CAD build for the part. Positions are in the model's coordinates, mm. Face numbers are marked on the shaded views. A direction names the side the tool comes from. Coordinates: 2 decimals unless noted, no trailing zeros. Loops run counter-clockwise (first coordinate to the right, second up) from the corner with the lowest first, then second, coordinate; pieces in that order, holes last. Notation, with made-up numbers: (21.5, 72) - (28.5, 72) arc R12 ccw to (28.5, 76) - close; hole circle Ø10 at (49.5, 56). An arc over 180 degrees is marked (long way). Put each result on its own line as item: value.
```python
from build123d import *

# Parameters (mm, degrees)
SKETCH1_W             = 4.45
SKETCH1_H             = 6
BOSS_EXTRUDE1_DEPTH   = 7.5
BOSS_EXTRUDE1_2_DEPTH = 7.5
SKETCH2_W             = 6.25
SKETCH2_H             = 6
SKETCH2_R             = 1.75
SKETCH2_W_2           = 4.260679938
SKETCH2_W_3           = 0.189320062
SKETCH2_W_4           = 7.55
BOSS_EXTRUDE2_DEPTH   = 3
SKETCH3_W             = 4
SKETCH3_H             = 1
CUT_EXTRUDE1_DEPTH    = 5


with BuildPart() as part:
    # Sketch1 → Boss-Extrude1 (new body)
    with BuildSketch(Plane.XY):
        with Locations((-3.775, -1.877941176)):
            Rectangle(SKETCH1_W, SKETCH1_H)
    extrude(amount=BOSS_EXTRUDE1_DEPTH)



with BuildPart() as body_2:
    # Sketch1 → Boss-Extrude1 2 (new body)
    with BuildSketch(Plane.XY):
        with Locations((3.775, -1.877941176)):
            Rectangle(SKETCH1_W, SKETCH1_H)
    extrude(amount=BOSS_EXTRUDE1_2_DEPTH)


with BuildPart() as part_1:
    add(part.part)

    add(body_2.part)  # Boss-Extrude2 merges body 2
    # Sketch2 → Boss-Extrude2 (add)
    # profile 1 of 5: a face of its own
    with BuildSketch(Plane(origin=(0, 0, 0), x_dir=(-1, 0, 0), z_dir=(0, 0, -1))):
        with Locations((-9.125, -1.877941176)):
            Rectangle(SKETCH2_W, SKETCH2_H)
        with Locations((-9.030339969, -1.877941176)):
            Circle(SKETCH2_R, mode=Mode.SUBTRACT)
    # profile 2 of 5: a face of its own
    with BuildSketch(Plane(origin=(0, 0, 0), x_dir=(-1, 0, 0), z_dir=(0, 0, -1))):
        with Locations((-3.680339969, -1.877941176)):
            Rectangle(SKETCH2_W_2, SKETCH2_H)
    # profile 3 of 5: a face of its own
    with BuildSketch(Plane(origin=(0, 0, 0), x_dir=(-1, 0, 0), z_dir=(0, 0, -1))):
        with Locations((-5.905339969, -1.877941176)):
            Rectangle(SKETCH2_W_3, SKETCH2_H)
    # profile 4 of 5: a face of its own
    with BuildSketch(Plane(origin=(0, 0, 0), x_dir=(-1, 0, 0), z_dir=(0, 0, -1))):
        with Locations((2.225, -1.877941176)):
            Rectangle(SKETCH2_W_4, SKETCH2_H)
    # profile 5 of 5: a face of its own
    with BuildSketch(Plane(origin=(0, 0, 0), x_dir=(-1, 0, 0), z_dir=(0, 0, -1))):
        with Locations((9.125, -1.877941176)):
            Rectangle(SKETCH2_W, SKETCH2_H)
        with Locations((9.030339969, -1.877941176)):
            Circle(SKETCH2_R, mode=Mode.SUBTRACT)
    extrude(amount=BOSS_EXTRUDE2_DEPTH)

    # Sketch3 → Cut-Extrude1 (cut)
    with BuildSketch(Plane.XY.offset(7.5)):
        with Locations((0, -1.877941176)):
            Rectangle(SKETCH3_W, SKETCH3_H)
    extrude(amount=-CUT_EXTRUDE1_DEPTH, mode=Mode.SUBTRACT)


solid = part_1.part
```
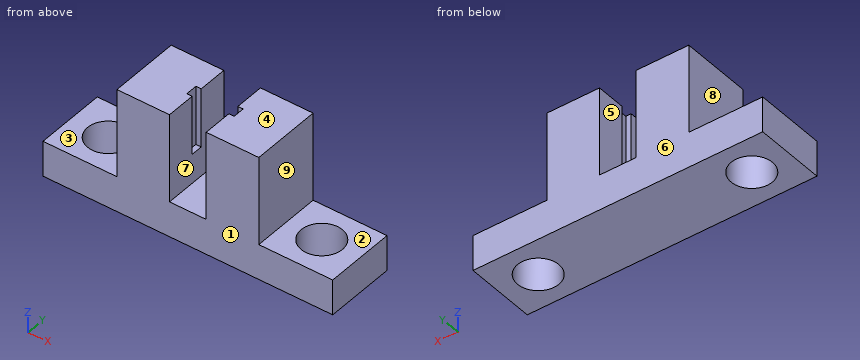
Q1. Slice it at C-C, the plane y = 0.2. Give the cut face in (x, z).
Determined:
outline: (-12.25, -3) - (12.25, -3) - (12.25, 0) - (6, 0) - (6, 7.5) - (1.55, 7.5) - (1.55, 0) - (-1.55, 0) - (-1.55, 7.5) - (-6, 7.5) - (-6, 0) - (-12.25, 0) - close
Q2. Wall check: L1, parallel to X at y = -4.25, z = 1.75; L2, parallel to Y at x = -1.75, z = 6.5; L3, parallel to X at y = -2, z = 3.5. Give the ranges that are in metal, low to high. Write a range as from..to.
Determined:
L1: -6..-1.55, 1.55..6
L2: -4.88..-2.38, -1.38..1.12
L3: -6..-2, 2..6
Q3. Mould opens along X. For the marked faces 6, 7, 8 and 9 say: +X half, -X half, draft (parallel to the pull), parting line (faces both ways), or undercut.
Determined:
face 6: draft
face 7: undercut
face 8: -X half
face 9: +X half
Q4. Slice it at B-B, the plane x = -9. Give the cut face in (y, z), then the cut area to 3 significant figures.
Determined:
outline: (-4.88, -3) - (-3.63, -3) - (-3.63, 0) - (-4.88, 0) - close; (-0.13, -3) - (1.12, -3) - (1.12, 0) - (-0.13, 0) - close
area: 7.50 mm2
Q5. Tool access for the marked faces 1, 2, 3, 4 and 5: list every direction of +Z, -Z, +X, -X, +Y, -Y with a clear straight run to the whole face (end or side of a thin tool).
Determined:
face 1: +Z, -Z, +X, -X, -Y
face 2: +Z, +X, +Y, -Y
face 3: +Z, -X, +Y, -Y
face 4: +Z, +X, -X, +Y, -Y
face 5: +Z, +Y, -Y
Q6. Pin check, flat tips, straight feed: pin 1 Ø3 at (y, z) = (-2.5, 5) entering from +X; pin 2 Ø2.5 at (x, y) = (0, -0.5) entering from +Z; pin 3 Ø3 at (y, z) = (-2, 4.5) entering from -X; pin 4 Ø3 at (x, y) = (9.03, -1.88) entering from -Z. Stop position of each tip, or through.
Determined:
pin 1: x = 6
pin 2: z = 0
pin 3: x = -6
pin 4: through
Q7. Slice it at D-D, the plane y = -3.2. Give the cut face in (x, z).
Determined:
outline: (-12.25, -3) - (-10.18, -3) - (-10.18, 0) - (-12.25, 0) - close; (-7.88, -3) - (7.88, -3) - (7.88, 0) - (6, 0) - (6, 7.5) - (1.55, 7.5) - (1.55, 0) - (-1.55, 0) - (-1.55, 7.5) - (-6, 7.5) - (-6, 0) - (-7.88, 0) - close; (10.18, -3) - (12.25, -3) - (12.25, 0) - (10.18, 0) - close
Q8. Slice it at A-A, the plane z = 2.25. Give the cut face in (x, y), then the cut area to 3 significant figures.
Determined:
outline: (-6, -4.88) - (-1.55, -4.88) - (-1.55, 1.12) - (-6, 1.12) - close; (1.55, -4.88) - (6, -4.88) - (6, 1.12) - (1.55, 1.12) - close
area: 53.4 mm2
